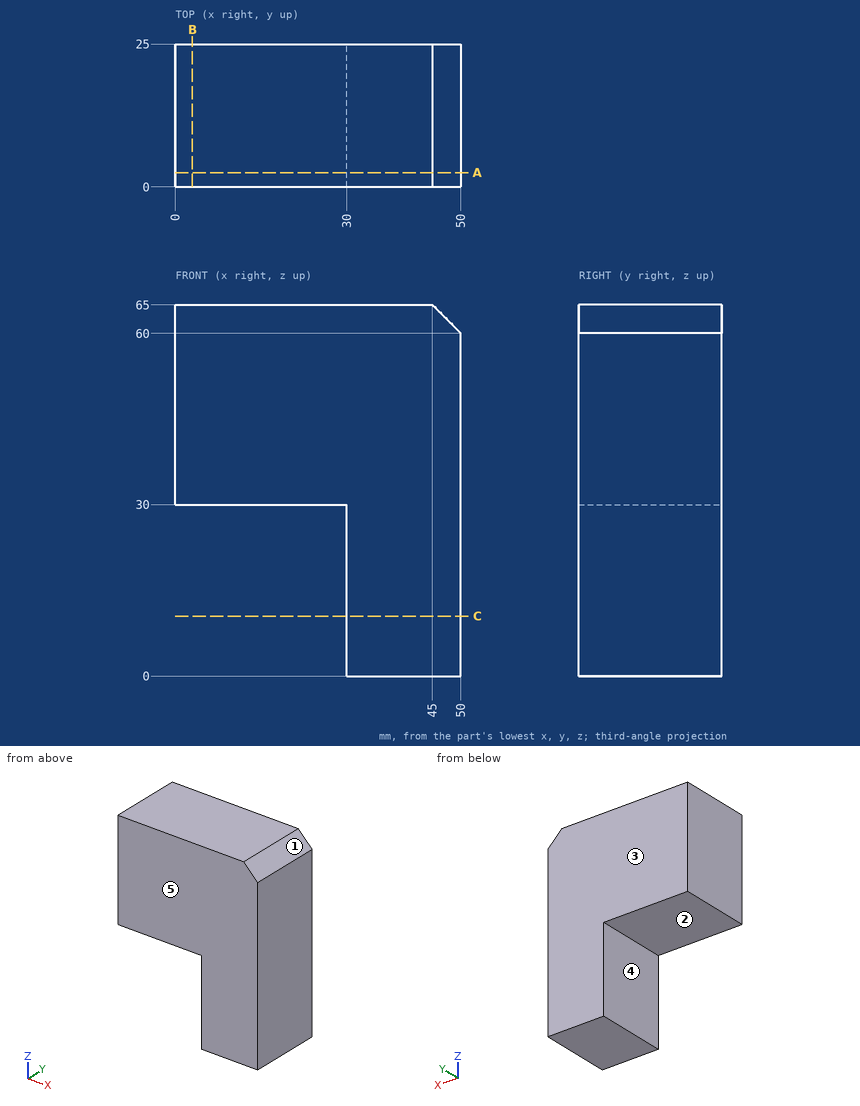
Answer from the drawing. Dimensions are ordinates in mm from the lowest x, y and z of the part. A direction names the side the tool comes from. Round coordinates to 2 decimals unless told otherwise and drop trailing zeros. Loops run counter-clockwise (first coordinate to the right, second up) from the corner with the lowest first, then second, coordinate; pieces in that order, holes last. Notation, with made-up numbers: (34, 11.5) - (80, 11.5) arc R15 cw to (80, 37.5) - close; hole circle Ø6 at (58.5, 22.5). An arc over 180 degrees is marked (long way). Return JSON: item names as keys, results as strings. Group by question number.
1. The part is cut by section A-A on y = 2.5. Determine the outline of the cut face in (x, z), then the cut area to 3 significant figures.
2. Which of the six approach directions +Z, -Z, +X, -X, +Y, -Y give full straight-line access (tool end or side, diameter ignored) to the marked faces 1 and 2?
3. The part is cut by section C-C on z = 10.5. Determine the outline of the cut face in (x, y), then the cut area to 3 significant figures.
4. The part is cut by section B-B on x = 3. Determine the outline of the cut face in (y, z).
5. Consider probe 1 along X at (y, z) = (14.25, 14.5); probe 2 along Z at (x, y) = (12, 14.75); probe 3 along X at (y, z) = (22.5, 62). Determine where each line is inside the solid, lowest interval first.
6. The mould has two halves that part along Y. Classify the marked faces 3, 4 and 5: pulls with the +Y half, pulls with the -Y half, needs draft (parallel to the pull), parting line crosses it, or undercut.
7. This flat-tipped pin is pushed along its axis until it touches: P1, Ø7.5, axis at y = 15.5, z = 15, coming from the -X side. Where does it stop, or does it pass through?
Resolved:
{
 "1": {"outline": "(0, 30) - (30, 30) - (30, 0) - (50, 0) - (50, 60) - (45, 65) - (0, 65) - close", "area": "2,340 mm²"},
 "2": {"face 1": "+Z, +X, +Y, -Y", "face 2": "-Z, -X, +Y, -Y"},
 "3": {"outline": "(30, 0) - (50, 0) - (50, 25) - (30, 25) - close", "area": "500 mm²"},
 "4": {"outline": "(0, 30) - (25, 30) - (25, 65) - (0, 65) - close"},
 "5": {"probe 1": "x = 30 to 50", "probe 2": "z = 30 to 65", "probe 3": "x = 0 to 48"},
 "6": {"face 3": "pulls with the +Y half", "face 4": "needs draft", "face 5": "pulls with the -Y half"},
 "7": {"P1": "stops at x = 30"}
}
